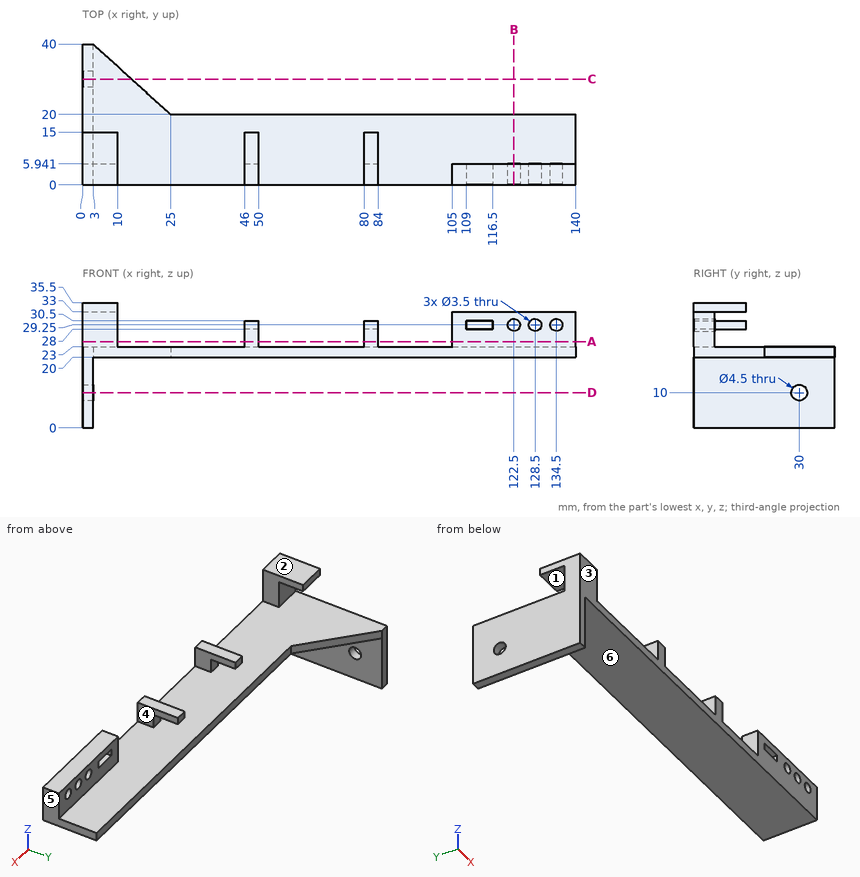
Source: three-view drawing plus pictorial views. Frame: mm from the lowest corner of the part. A direction names the side the tool comes from. Round coordinates to 2 decimals unless told otherwise and drop trailing zeros. Loops run counter-clockwise (first coordinate to the right, second up) from the corner with the lowest first, then second, coordinate; pieces in that order, holes last.
Item 1: Section D-D, the plane z = 10. Output: boundary loops of the cut face in (x, y).
Checked values:
outline: (0, 0) - (3, 0) - (3, 27.75) - (0, 27.75) - close; (0, 32.25) - (3, 32.25) - (3, 40) - (0, 40) - close
Item 2: Section C-C, the plane y = 30. Output: boundary loops of the cut face in (x, z).
Checked values:
outline: (0, 0) - (3, 0) - (3, 7.75) - (0, 7.75) - close; (0, 12.25) - (3, 12.25) - (3, 20) - (14, 20) - (14, 23) - (0, 23) - close
Item 3: Section A-A, the plane z = 24.5. Output: boundary loops of the cut face in (x, y).
Checked values:
outline: (0, 0) - (10, 0) - (10, 5.94) - (0, 5.94) - close; (46, 0) - (50, 0) - (50, 5.94) - (46, 5.94) - close; (80, 0) - (84, 0) - (84, 5.94) - (80, 5.94) - close; (105, 0) - (140, 0) - (140, 5.94) - (105, 5.94) - close
Item 4: Section B-B, the plane x = 122.5. Output: boundary loops of the cut face in (y, z).
Checked values:
outline: (0, 20) - (20, 20) - (20, 23) - (5.94, 23) - (5.94, 27.5) - (0, 27.5) - close; (0, 31) - (5.94, 31) - (5.94, 33) - (0, 33) - close
Item 5: Mould query, pull axis Z, two halves, no side actions, for the marked faces 1, 2 and 3. Classes: released by +Z, released by -Z, zero draft, split by the parting line, or undercut.
Checked values:
face 1: undercut
face 2: released by +Z
face 3: zero draft
Item 6: Reachability of the marked faces 4, 5 and 6 from +Z, -Z, +X, -X, +Y, -Y: full face, straight path, thin tool, end or side. Return the list, or none.
Checked values:
face 4: +Z, +Y, -Y
face 5: +Z, -Z, +X, +Y, -Y
face 6: -Z, +X, +Y, -Y
Item 7: Line query: L1, parallel to Y at x = 1, z = 10; L2, parallel to Y at x = 117, z = 29; L3, parallel to Z at x = 134.5, y = 1.55. Output: solid intervals per line, ascending.
Checked values:
L1: y = 0 to 27.75, 32.25 to 40
L2: y = 0 to 5.94
L3: z = 20 to 27.5, 31 to 33
Item 8: Contact query for flat-ended pins moving along their axis: P1, Ø5.5, axis at x = 122.5, z = 29.25, coming from the +Y side; P2, Ø3, axis at y = 25, z = 10.5, coming from the +X side; P3, Ø8, axis at x = 63.5, y = 25.5, coming from the +Z side; P4, Ø6.5, axis at x = 111.5, y = 2, coming from the +Z side. Output: stop coordinate, or through.
Checked values:
P1: stops at y = 5.94
P2: stops at x = 3
P3: passes through
P4: stops at z = 33
